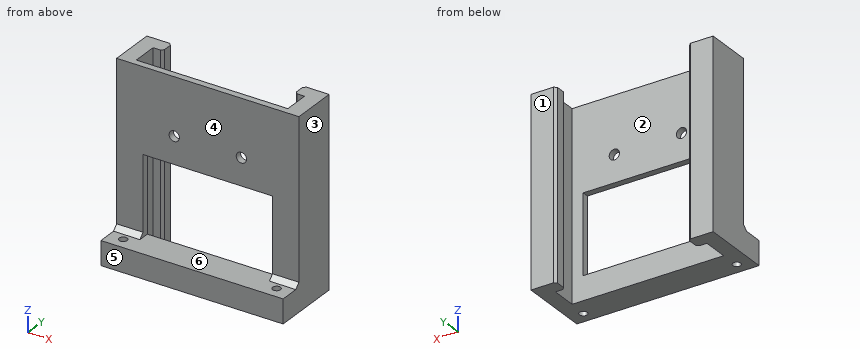
from build123d import *

# Parameters (mm, degrees)
EXTRUDE_1_DEPTH      = 39
HOLE_WIZARD_M4_1_D   = 4.3
CHAMFER_1_SIZE       = 1
SKETCH_8_W           = 76
SKETCH_8_H           = 10
EXTRUDE_2_DEPTH      = 10
CUT_EXTRUDE_2_REACH  = 59.705
SKETCH_9_W           = 54
SKETCH_9_H           = 33
CHAMFER_2_SIZE       = 2
HOLE_WIZARD_M4_1_2_D = 3.3


with BuildPart() as part:
    # 草图1 → 凸台-拉伸1 (new, symmetric)
    with BuildSketch(Plane.XY):
        Polygon((-27.5, 19.1), (-38, 19.1), (-38, 0), (38, 0), (38, 19.1), (27.5, 19.1), (27.5, 13.3), (31.6, 13.3), (31.6, 2.7), (-31.6, 2.7), (-31.6, 13.3), (-27.5, 13.3), align=None)
    extrude(amount=EXTRUDE_1_DEPTH, both=True)

    # Hole Wizard M4 _1 (through all)
    with Locations(Plane(origin=(0, 0, 0), x_dir=(-1, 0, 0), z_dir=(0, -1, 0))):
        with Locations((-14, -15.3), (14, -15.3)):
            Hole(HOLE_WIZARD_M4_1_D / 2)

    # 倒角1
    chamfer_1_edges = [part.edges().sort_by_distance(p)[0] for p in [
        (-27.5, 13.3, 0),
        (27.5, 13.3, 0),
        (27.5, 19.1, 0),
        (-27.5, 19.1, 0),
    ]]
    chamfer(chamfer_1_edges, length=CHAMFER_1_SIZE)

    # 草图8 → 凸台-拉伸2 (add)
    with BuildSketch(Plane.XZ):
        with Locations((0, -34)):
            Rectangle(SKETCH_8_W, SKETCH_8_H)
    extrude(amount=EXTRUDE_2_DEPTH)

    # 草图9 → 切除-拉伸2 (cut, up to next)
    with BuildSketch(Plane.XZ, mode=Mode.PRIVATE) as cut_extrude_2_sk1:
        with Locations((0, -12.5)):
            Rectangle(SKETCH_9_W, SKETCH_9_H)
    cut_extrude_2_tool1 = extrude(cut_extrude_2_sk1.sketch, amount=-CUT_EXTRUDE_2_REACH, mode=Mode.PRIVATE) & part.part
    add(cut_extrude_2_tool1.solids().sort_by_distance((0, 0, -12.5))[0], mode=Mode.SUBTRACT)

    # 倒角2
    chamfer_2_edges = [part.edges().sort_by_distance(p)[0] for p in [
        (32.5, 0, -29),
        (-32.5, 0, -29),
    ]]
    chamfer(chamfer_2_edges, length=CHAMFER_2_SIZE)

    # Hole Wizard M4 _1 2 (through all)
    with Locations(Plane(origin=(0, 0, -39), x_dir=(-1, 0, 0), z_dir=(0, 0, -1))):
        with Locations((32, -5), (-32, -5)):
            Hole(HOLE_WIZARD_M4_1_2_D / 2)


solid = part.part
Can you work these out from the model? Positions are in its coordinate system, mm. Face numbers are marked on the shaded views. A direction names the side the tool comes from. Coordinates: 2 decimals unless noted, no trailing zeros. Loops run counter-clockwise (first coordinate to the right, second up) from the corner with the lowest first, then second, coordinate; pieces in that order, holes last. Notation, with made-up numbers: M 3.25,-32 L 23.25,-32 A17 ccw 23.25,0 Z; hole C 42.5,3.25 d2. An arc over 180 degrees is marked long. Return JSON: item names as keys, results as strings. Group by question number.
Item 1: If I drill on L1, parallel to X at y = 0.85, z = 15.3; L2, parallel to Y at x = -32, z = -33.25; L3, parallel to X at y = 3.5, z = 17.5, over which ranges is the centre line in solid material (lowest first)? Write a range as from..to.
Item 2: Imagine slicing it at D-D (y = -5). Please give me the cut outline in (x, z).
Item 3: Imagine slicing it at C-C (z = -30). Please give me the cut outline in (x, y).
Item 4: Imagine slicing it at A-A (y = 7.5). Please give me the cut outline in (x, z).
Item 5: I'm going to push flat-ended pins straight in: pin 1 Ø3.5 at (x, z) = (-29.5, 15) entering from -Y; pin 2 Ø7 at (x, z) = (-14, 15.3) entering from +Y; pin 3 Ø3.5 at (x, z) = (14, 15.3) entering from +Y. Where does each tip first touch, or does it pass through?
Item 6: On a 3-axis mill with a long thin cutter (end or side, diameter ignored), from which of +Z, -Z, +X, -X, +Y, -Y can I reach the whole of each face in a straight line? I mean the marked faces 4, 5 and 6. Say none if no direction works.
Item 7: Imagine slicing it at B-B (x = 9). Please give me the cut outline in (y, z), and give its area (4 significant figures).
Item 8: Thinking about a two-plate mould opening in X: for the marked faces 1, 2 and 3, which applies, released by +X, released by -X, zero draft, split by the parting line, or undercut?
Verdict:
{
 "1": {"L1": "x = -38..-16.15, -11.85..11.85, 16.15..38", "L2": "y = -10..-6.65, -3.35..19.1", "L3": "x = -38..-31.6, 31.6..38"},
 "2": {"outline": "M -38,-39 L -33.65,-39 L -33.65,-29 L -38,-29 Z; M -30.35,-39 L 30.35,-39 L 30.35,-29 L -30.35,-29 Z; M 33.65,-39 L 38,-39 L 38,-29 L 33.65,-29 Z"},
 "3": {"outline": "M -38,-10 L 38,-10 L 38,19.1 L 28.5,19.1 L 27.5,18.1 L 27.5,14.3 L 28.5,13.3 L 31.6,13.3 L 31.6,2.7 L -31.6,2.7 L -31.6,13.3 L -28.5,13.3 L -27.5,14.3 L -27.5,18.1 L -28.5,19.1 L -38,19.1 Z; hole C -32,-5 d3.3; hole C 32,-5 d3.3"},
 "4": {"outline": "M -38,-39 L -31.6,-39 L -31.6,39 L -38,39 Z; M 31.6,-39 L 38,-39 L 38,39 L 31.6,39 Z"},
 "5": {"pin 1": "stops at y = 0", "pin 2": "stops at y = 2.7", "pin 3": "passes through"},
 "6": {"face 4": "+Z, +X, -X, -Y", "face 5": "+Z, -Z, +X, -X, -Y", "face 6": "-Y"},
 "7": {"outline": "M -10,-39 L 2.7,-39 L 2.7,-29 L -10,-29 Z; M 0,4 L 2.7,4 L 2.7,39 L 0,39 Z", "area": "221.5 mm^2"},
 "8": {"face 1": "zero draft", "face 2": "undercut", "face 3": "released by +X"}
}
